For this review, take the finished solid that the model builds, in its own axes (mm). Face numbers are marked on the shaded views. A direction names the side the tool comes from. Give positions to 0.01 mm unless a question says otherwise; leave off trailing zeros. Write each loop counter-clockwise with the first axis right and the second up, starting at its lowest first coordinate (ties: lowest second). Pieces come first, ordered by that corner, then holes.
from build123d import *

# Parameters (mm, degrees)
SKETCH2_R           = 40
BOSS_EXTRUDE1_DEPTH = 25
SKETCH3_R           = 27.5
CUT_EXTRUDE1_DEPTH  = 17
CUT_EXTRUDE3_DEPTH  = 9
SKETCH5_R           = 4
BOSS_EXTRUDE3_DEPTH = 25
SKETCH6_R           = 2.5
CUT_EXTRUDE4_DEPTH  = 10
SKETCH18_R          = 48
SKETCH18_R_2        = 40
BOSS_EXTRUDE5_DEPTH = 25


with BuildPart() as part:
    # Sketch2 → Boss-Extrude1 (new body)
    with BuildSketch(Plane(origin=(0, 0, 0), x_dir=(1, 0, 0), z_dir=(0, 1, 0))):
        with Locations((-41.86871729, 18.12498584)):
            Circle(SKETCH2_R)
    extrude(amount=BOSS_EXTRUDE1_DEPTH)

    # Sketch3 → Cut-Extrude1 (cut)
    with BuildSketch(Plane.XZ):
        with Locations((-41.345752459, -18.274404363)):
            Circle(SKETCH3_R)
    extrude(amount=-CUT_EXTRUDE1_DEPTH, mode=Mode.SUBTRACT)

    # Sketch4 → Cut-Extrude3 (cut, through all)
    with BuildSketch(Plane.XZ.offset(-17)):
        with BuildLine():
            ThreePointArc((-14.70636998, -22.421133954), (-15.889488047, -9.10669066), (-23.210546195, 2.077059883))
            add(Edge.make_bspline(
                [(-23.210546195, 2.077059883), (-46.355723427, -18.546490673), (-14.70636998, -22.421133954)],
                knots=[0, 0, 0, 1, 1, 1], degree=2))
        make_face()
        with BuildLine():
            ThreePointArc((-35.453936971, -44.866350679), (-23.423134112, -38.521320345), (-15.904630116, -27.18678352))
            add(Edge.make_bspline(
                [(-15.904630116, -27.18678352), (-43.876407216, -14.328885453), (-35.453936971, -44.866350679)],
                knots=[0, 0, 0, 1, 1, 1], degree=2))
        make_face()
        with BuildLine():
            ThreePointArc((-64.70739494, -33.443105934), (-54.300273107, -42.654690689), (-40.717881586, -45.600894873))
            add(Edge.make_bspline(
                [(-40.717881586, -45.600894873), (-36.156523784, -13.602103875), (-64.70739494, -33.443105934)],
                knots=[0, 0, 0, 1, 1, 1], degree=2))
        make_face()
        with BuildLine():
            ThreePointArc((-62.550469834, 0), (-68.986764274, -13.557543689), (-67.346528808, -28.475402269))
            add(Edge.make_bspline(
                [(-67.346528808, -28.475402269), (-35.360422095, -20.710055245), (-62.550469834, 0)],
                knots=[0, 0, 0, 1, 1, 1], degree=2))
        make_face()
        with BuildLine():
            ThreePointArc((-26.174469517, 4.456878273), (-41.880660096, 9.375011567), (-57.58257302, 4.44323824))
            add(Edge.make_bspline(
                [(-57.58257302, 4.44323824), (-43.38243666, -25.570584632), (-26.174469517, 4.456878273)],
                knots=[0, 0, 0, 1, 1, 1], degree=2))
        make_face()
    extrude(amount=-CUT_EXTRUDE3_DEPTH, mode=Mode.SUBTRACT)

    # Sketch5 → Boss-Extrude3 (add)
    with BuildSketch(Plane.XZ.offset(-17)):
        with Locations((-41.86871729, -18.12498584)):
            Circle(SKETCH5_R)
    extrude(amount=BOSS_EXTRUDE3_DEPTH)

    # Sketch6 → Cut-Extrude4 (cut)
    with BuildSketch(Plane.XZ.offset(8)):
        with Locations((-41.86871729, -18.12498584)):
            Circle(SKETCH6_R)
    extrude(amount=-CUT_EXTRUDE4_DEPTH, mode=Mode.SUBTRACT)

    # Sketch18 → Boss-Extrude5 (add)
    with BuildSketch(Plane(origin=(0, 0, 0), x_dir=(1, 0, 0), z_dir=(0, 1, 0))):
        with Locations((-41.86871729, 18.12498584)):
            Circle(SKETCH18_R)
        with Locations((-41.86871729, 18.12498584)):
            Circle(SKETCH18_R_2, mode=Mode.SUBTRACT)
    extrude(amount=BOSS_EXTRUDE5_DEPTH)


solid = part.part
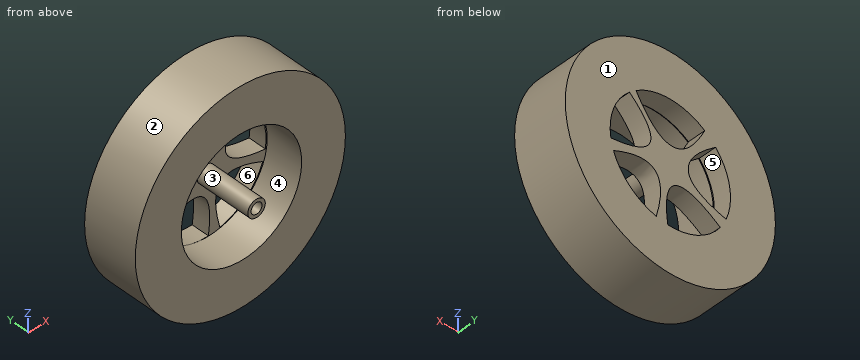
(1) We need section A-A (y = 6.5). Write out the cut boundary in (x, z), and give its area (3 significant figures).
(2) We need section C-C (y = -5). Write out the cut boundary in (x, z), and give its area (3 significant figures).
(3) For L1, parallel to Z at x = -23, y = 22; L2, parallel to X at y = 20, z = -33.5; L3, parallel to Y at x = -4.5, z = -19, list the stretches that pass through material, from the lowest coordinate up.
(4) The part is to be moulded in two halves that separate along Z. For the marked faces 1, 2 and 3, say which applies: +Z half, -Z half, draft (parallel to the pull), parting line (faces both ways), or undercut.
(5) Clearance check with flat-ended pins moving along their axes: pin 1 Ø2 at (x, z) = (-24, 19.5) entering from -Y; pin 2 Ø2 at (y, z) = (15, -55) entering from +X; pin 3 Ø3 at (x, z) = (-41.87, -18.12) entering from -Y. State where each tip first meets the part, or that it passes through.
(6) We need section B-B (x = -22). Count the separate pieces of the cut face and the enclosed holes in it, and give its area (3 significant figures).
(7) Tool access review of the marked faces 4, 5 and 6: name each direction out of +Z, -Z, +X, -X, +Y, -Y from which nothing blocks a thin tool from reaching the whole face with its end or side.
The answers:
1. outline: circle Ø96 at (-41.87, -18.12); circle Ø8 at (-41.87, -18.12); hole circle Ø55 at (-41.35, -18.27)
1. area: 4,910 mm2
2. outline: circle Ø8 at (-41.87, -18.12); hole circle Ø5 at (-41.87, -18.12)
2. area: 30.6 mm2
3. L1: z = -62.26 to -38.13, -24.44 to -20.87, 1.88 to 26.01
3. L2: x = -87.34 to -64.67, -40.39 to -37.4, -19.07 to 3.6
3. L3: y = 0 to 25
4. face 1: draft
4. face 2: parting line
4. face 3: undercut
5. pin 1: stops at y = 0
5. pin 2: stops at x = -9.98
5. pin 3: stops at y = 2
6. separate pieces: 3
6. enclosed holes: 0
6. area: 1,250 mm2
7. face 4: -Y
7. face 5: +Y
7. face 6: +Y, -Y
